from build123d import *

# Parameters (mm, degrees)
F0_W      = 58.57
F0_H      = 123.84
F1_DEPTH  = 7.67
F2_R      = 5.08
F3_R      = 5.08
F4_R      = 5.08
F5_R      = 5.08
F8_W      = 6.225877
F8_H      = 1.738168
F9_DEPTH  = 12.7
F10_R     = 1.719238
F11_DEPTH = 12.7
F7_R      = 5.45
F12_DEPTH = 0.1


with BuildPart() as f1:
    # F0 (on Front) → F1 (new body)
    with BuildSketch(Plane.XZ):
        with Locations((2.323339, -30.135072)):
            Rectangle(F0_W, F0_H)
    extrude(amount=F1_DEPTH)

    # F2
    f2_edges = [f1.edges().sort_by_distance(p)[0] for p in [
        (-26.961661, -3.835, 31.784928),
    ]]
    fillet(f2_edges, radius=F2_R)

    # F3
    f3_edges = [f1.edges().sort_by_distance(p)[0] for p in [
        (31.608339, -3.835, 31.784928),
    ]]
    fillet(f3_edges, radius=F3_R)

    # F4
    f4_edges = [f1.edges().sort_by_distance(p)[0] for p in [
        (31.608339, -3.835, -92.055072),
    ]]
    fillet(f4_edges, radius=F4_R)

    # F5
    f5_edges = [f1.edges().sort_by_distance(p)[0] for p in [
        (-26.961661, -3.835, -92.055072),
    ]]
    fillet(f5_edges, radius=F5_R)

    # F8 (on face) → F9 (cut)
    with BuildSketch(Plane(origin=(0, 0, -92.055072), x_dir=(1, 0, 0), z_dir=(0, 0, -1))):
        with Locations((-0.13871, 3.651316)):
            Rectangle(F8_W, F8_H)
    extrude(amount=-F9_DEPTH, mode=Mode.SUBTRACT)

    # F10 (on face) → F11 (cut)
    with BuildSketch(Plane(origin=(0, 0, -92.055072), x_dir=(1, 0, 0), z_dir=(0, 0, -1))):
        with Locations((9.932925, 4.50147)):
            Circle(F10_R)
    extrude(amount=-F11_DEPTH, mode=Mode.SUBTRACT)

    # F7 (on face) → F12 (cut)
    with BuildSketch(Plane.XZ.offset(7.67)):
        with Locations((-0.289605, -83.01686)):
            Circle(F7_R)
    extrude(amount=-F12_DEPTH, mode=Mode.SUBTRACT)


solid = f1.part
Could you check a few things on this model? Use its own coordinates, in mm. A direction names the side the tool comes from. Coordinates: 2 decimals unless noted, no trailing zeros. Order: outer loops, then holes, each group sorted by start corner. A loop starts at its lowest first (then second) coordinate and runs counter-clockwise, first axis right, second up. Notation, with made-up numbers: (61, -7) -> (85, -7) arc R21 ccw to (85, -1) -> close; hole circle Ø7 at (-5.75, -16.5). An arc over 180 degrees is marked (long way). One line per item, written item: value. Start each with the question number.
1) I'm going to push flat-ended pins straight in: pin 1 (5 mm diameter, centred on x = -1.5, z = -87.5, fed in from +Y); pin 2 (5.5 mm diameter, centred on x = -1, z = -81, fed in from -Y); pin 3 (1 mm diameter, centred on x = 10.5, y = -4.5, fed in from -Z). Where does each tip first touch, or does it pass through?
2) Imagine slicing it at A-A on x = 0. List the corners of the cut face in (y, z) for me.
3) We'd pull the mould along X, two halves only. Please class faces 1 (the cylindrical face through (30.081, -3.889, 30.336)), 2 (the flat face through (2, -7.67, -29)), 3 (the flat face through (0, -4.52, -86)): +X half, -X half, draft (parallel to the pull), parting line (faces both ways), or undercut.
4) Which directions (+Z, -Z, +X, -X, +Y, -Y) give clear straight access to the entire face, cutting with the end or side of a thin tool? Please do faces 4 (the flat face through (0, -7.57, -83)), 5 (the flat face through (2, -5, -92.055)), 6 (the flat face through (0, -2.782, -86)).
5) If I drill on L1, parallel to Z at x = 11.5, y = -4.75; L2, parallel to Z at x = -23.5, y = -1.75, over which ranges is the centre line in solid material (lowest first)? Write a range as [from, to].
Answer list:
1. pin 1: stops at y = 0
1. pin 2: stops at y = -7.57
1. pin 3: stops at z = -79.36
2. outline: (-7.67, -92.06) -> (-4.52, -92.06) -> (-4.52, -79.36) -> (-2.78, -79.36) -> (-2.78, -92.06) -> (0, -92.06) -> (0, 31.78) -> (-7.67, 31.78) -> (-7.67, -77.57) -> (-7.57, -77.57) -> (-7.57, -88.46) -> (-7.67, -88.46) -> close
3. face 1: +X half
3. face 2: draft
3. face 3: undercut
4. face 4: -Y
4. face 5: -Z, +X, -X, +Y, -Y
4. face 6: -Z
5. L1: z = [-79.36, 31.78]
5. L2: z = [-91.79, 31.52]
